```python
from build123d import *

# Parameters (mm, degrees)
SKETCH1_W           = 2.92
SKETCH1_H           = 2.92
BOSS_EXTRUDE1_DEPTH = 3


with BuildPart() as part:
    # Sketch1 → Boss-Extrude1 (new body)
    with BuildSketch(Plane.XY):
        with BuildLine():
            Line((28.134570185, 8.537968033), (22.134570185, 14.537968033))
            Line((22.134570185, 14.537968033), (-27.865429815, 14.537968033))
            Line((-27.865429815, 14.537968033), (-33.865429815, 8.537968033))
            Line((-33.865429815, 8.537968033), (-33.865429815, -20.462031967))
            Line((-33.865429815, -20.462031967), (-28.865429815, -25.462031967))
            Line((-28.865429815, -25.462031967), (-26.045429815, -25.462031967))
            Line((-26.045429815, -25.462031967), (-26.045429815, -20.462031967))
            ThreePointArc((-26.045429815, -20.462031967), (-25.845429815, -18.962031967), (-26.045429815, -17.462031967))
            Line((-26.045429815, -17.462031967), (-26.045429815, -12.462031967))
            ThreePointArc((-26.045429815, -12.462031967), (-25.845429815, -10.962031967), (-26.045429815, -9.462031967))
            Line((-26.045429815, -9.462031967), (-26.045429815, -4.462031967))
            Line((-26.045429815, -4.462031967), (-20.045429815, -4.462031967))
            Line((-20.045429815, -4.462031967), (-20.045429815, -9.462031967))
            ThreePointArc((-20.045429815, -9.462031967), (-20.245429815, -10.962031967), (-20.045429815, -12.462031967))
            Line((-20.045429815, -12.462031967), (-20.045429815, -17.462031967))
            ThreePointArc((-20.045429815, -17.462031967), (-20.245429815, -18.962031967), (-20.045429815, -20.462031967))
            Line((-20.045429815, -20.462031967), (-20.045429815, -25.462031967))
            Line((-20.045429815, -25.462031967), (14.314570185, -25.462031967))
            Line((14.314570185, -25.462031967), (14.314570185, -20.462031967))
            ThreePointArc((14.314570185, -20.462031967), (14.514570185, -18.962031967), (14.314570185, -17.462031967))
            Line((14.314570185, -17.462031967), (14.314570185, -12.462031967))
            ThreePointArc((14.314570185, -12.462031967), (14.514570185, -10.962031967), (14.314570185, -9.462031967))
            Line((14.314570185, -9.462031967), (14.314570185, -4.462031967))
            Line((14.314570185, -4.462031967), (20.314570185, -4.462031967))
            Line((20.314570185, -4.462031967), (20.314570185, -9.462031967))
            ThreePointArc((20.314570185, -9.462031967), (20.164790454, -10.20539467), (20.114570185, -10.962031967))
            ThreePointArc((20.114570185, -10.962031967), (20.164790454, -11.718669265), (20.314570185, -12.462031967))
            Line((20.314570185, -12.462031967), (20.314570185, -17.462031967))
            ThreePointArc((20.314570185, -17.462031967), (20.164790454, -18.20539467), (20.114570185, -18.962031967))
            ThreePointArc((20.114570185, -18.962031967), (20.164790454, -19.718669265), (20.314570185, -20.462031967))
            Line((20.314570185, -20.462031967), (20.314570185, -25.462031967))
            Line((20.314570185, -25.462031967), (23.134570185, -25.462031967))
            Line((23.134570185, -25.462031967), (28.134570185, -20.462031967))
            Line((28.134570185, -20.462031967), (28.134570185, 8.537968033))
        make_face()
        with Locations((-23.405429815, 7.077968033)):
            Rectangle(SKETCH1_W, SKETCH1_H, mode=Mode.SUBTRACT)
        with Locations((17.674570185, 7.077968033)):
            Rectangle(SKETCH1_W, SKETCH1_H, mode=Mode.SUBTRACT)
    extrude(amount=BOSS_EXTRUDE1_DEPTH)


solid = part.part
```
Could you check a few things on this model? Use its own coordinates, in mm. A direction names the side the tool comes from. Round coordinates to 2 decimals unless told otherwise and drop trailing zeros. Loops run counter-clockwise (first coordinate to the right, second up) from the corner with the lowest first, then second, coordinate; pieces in that order, holes last. Notation, with made-up numbers: (16.25, 3) - (50.25, 3) arc R34 ccw to (50.25, 36) - close; hole circle Ø10 at (47, -16). An arc over 180 degrees is marked (long way). Answer in a Markdown table with one row per item. Add a question column.
(1) If we section it at C-C (z = 2.3): State how many separate pieces and enclosed holes the cut face has, plus the area to 3 significant figures.
(2) If we mould it in two halves opening along Y, with no side actions, what happens to faces 4 (the face through (-24.865, 7, 1)), 5 (the face through (-26.045, -23, 1)), 6 (the face through (25.177, 11.496, 1.479)), 7 (the face through (25.6, -22.997, 1.479))? For each: pulls with the +Y half, pulls with the -Y half, needs draft (parallel to the pull), parting line crosses it, or undercut.
(3) If we section it at D-D (y = 12): Please give me the cut outline in (x, z), plus the area to 3 significant figures.
(4) I need wall thicknesses on line 1 along X through (y, z) = (-6, 2.2); line 2 along X through (y, z) = (-9.5, 0.2); line 3 along Y through (x, z) = (-25.5, 2.05). Which ranges of each line are inside material? Lowest first, please.
(5) For faces 1 (the face through (-20.045, -23, 1)), 2 (the face through (20.315, -7, 1)), 3 (the face through (-3, -5, 0)), which set-ups out of +Z, -Z, +X, -X, +Y, -Y let a thin tool reach every point of the face, with its end or its side?
(6) I'm going to push a flat-ended pin straight in: pin 1 (1.5 mm diameter, centred on x = 17.5, z = 1.5, fed in from -Y). Where does the tip first touch, or does it pass through?
(7) If we section it at A-A (x = -23): Please give me the cut outline in (y, z), plus the area to 3 significant figures.
(8) If we section it at B-B (y = -15.5): Please give me the cut outline in (x, z).
Model answer:
| question | item | result |
|---|---|---|
| 1 | separate pieces | 1 |
| 1 | enclosed holes | 2 |
| 1 | area | 2,150 mm² |
| 2 | face 4 | undercut |
| 2 | face 5 | needs draft |
| 2 | face 6 | pulls with the +Y half |
| 2 | face 7 | pulls with the -Y half |
| 3 | outline | (-30.4, 0) - (24.67, 0) - (24.67, 3) - (-30.4, 3) - close |
| 3 | area | 165 mm² |
| 4 | line 1 | x = -33.87 to -26.05, -20.05 to 14.31, 20.31 to 28.13 |
| 4 | line 2 | x = -33.87 to -26.04, -20.06 to 14.32, 20.3 to 28.13 |
| 4 | line 3 | y = -4.46 to 14.54 |
| 5 | face 1 | +Z, -Z, -Y |
| 5 | face 2 | +Z, -Z |
| 5 | face 3 | -Z, +X, -X, +Y, -Y |
| 6 | pin 1 | stops at y = -4.46 |
| 7 | outline | (-4.46, 0) - (5.62, 0) - (5.62, 3) - (-4.46, 3) - close; (8.54, 0) - (14.54, 0) - (14.54, 3) - (8.54, 3) - close |
| 7 | area | 48.2 mm² |
| 8 | outline | (-33.87, 0) - (-26.05, 0) - (-26.05, 3) - (-33.87, 3) - close; (-20.05, 0) - (14.31, 0) - (14.31, 3) - (-20.05, 3) - close; (20.31, 0) - (28.13, 0) - (28.13, 3) - (20.31, 3) - close |
